Build history of the part. All positions in model axes, mm. A direction names the side the tool comes from. Give positions to 0.01 mm unless a question says otherwise; leave off trailing zeros. Write each loop counter-clockwise with the first axis right and the second up, starting at its lowest first coordinate (ties: lowest second). Pieces come first, ordered by that corner, then holes. Notation, with made-up numbers: (-32.75, -18.75) -> (-3.75, -18.75) arc R28 cw to (-3.75, 8.25) -> close; hole circle Ø10 at (-22, 25). An arc over 180 degrees is marked (long way). Put each result on its own line as item: value. Start each with the question number.
Item 1: Drill centre lines: line 1 along Y through (x, z) = (52.5, 7); line 2 along X through (y, z) = (9.5, 26.5). Where is each one in solid material? Low to high.
Item 2: Flat gauge pin, fed straight in: pin 1 Ø19 at (x, y) = (-20.5, 74) entering from +Z. Where does the tip first touch, or does it go through?
Item 3: Slice it at B-B, the plane z = 31.5. List the corners of the cut face in (x, y), plus the area to 3 significant figures.
Item 4: Slice it at C-C, the plane y = 63.5. List the corners of the cut face in (x, z), plus the area to 3 significant figures.
Item 5: Tool access for faces 1 (the cylindrical face through (-36.56, -3.39, 3.79)), 2 (the flat face through (82, -1, 25.4)), 3 (the flat face through (-1, 85.09, 15)), 4 (the flat face through (-1, -88.9, 14)): list every direction of +Z, -Z, +X, -X, +Y, -Y with a clear straight run to the whole face (end or side of a thin tool).
Item 6: Two-plate mould, pull along Y, no slides. Class faces 5 (the cylindrical face through (-87.372, 87.451, 14.13)), 6 (the cylindrical face through (-36.56, 3.39, 3.79)), 7 (the flat face through (-1, 20, 0)): pulls with the +Y half, pulls with the -Y half, needs draft (parallel to the pull), parting line crosses it, or undercut.
Item 7: Slice it at D-D, the plane z = 13. List the corners of the cut face in (x, y).
Item 8: Slice it at A-A, the plane x = -16. List the corners of the cut face in (y, z).
```python
from build123d import *

# Parameters (mm, degrees)
F0_W        = 177.8
F0_H        = 177.8
F0_W_2      = 170.18
F0_H_2      = 170.18
F1_DEPTH    = 25.4
F0_W_3      = 76.2
F0_H_3      = 9.652
F2_DEPTH    = 5.08
F3_T1_DEPTH = 5.08
F5_DEPTH    = 177.8
F6_W        = 78.74
F6_H        = 15.522254324
F7_DEPTH    = 177.801
F8_R        = 5.08
F9_R        = 2.54


# Not quite as in the source:
# - a fillet or chamfer that OpenCascade refuses, or shapes differently, is made with other operations: its cross-section is extruded or revolved along the edge and cut away or added


with BuildPart() as f1:
    # F0 (on Top) → F1 (new body)
    with BuildSketch(Plane.XY):
        Rectangle(F0_W, F0_H)
        Rectangle(F0_W_2, F0_H_2, mode=Mode.SUBTRACT)
    extrude(amount=F1_DEPTH)

    # F0 (on Top) → F2 (join)
    with BuildSketch(Plane.XY):
        Rectangle(F0_W_2, F0_H_2)
        Rectangle(F0_W_3, F0_H_3, mode=Mode.SUBTRACT)
    extrude(amount=F2_DEPTH)

    # F3: fillet of radius 5.08 on 4 edges, made by hand

    # F3_s2 → F3_t1 (join)
    with BuildSketch(Plane.XY):
        with BuildLine():
            ThreePointArc((33.02, 4.826), (36.6121024484, 3.3381024484), (38.1, -0.254))
            Line((38.1, -0.254), (38.1, 4.826))
            Line((38.1, 4.826), (33.02, 4.826))
        make_face()
        with BuildLine():
            ThreePointArc((38.1, 0.254), (36.6121024484, -3.3381024484), (33.02, -4.826))
            Line((33.02, -4.826), (38.1, -4.826))
            Line((38.1, -4.826), (38.1, 0.254))
        make_face()
        with BuildLine():
            ThreePointArc((-38.1, -0.254), (-36.6121024484, 3.3381024484), (-33.02, 4.826))
            Line((-33.02, 4.826), (-38.1, 4.826))
            Line((-38.1, 4.826), (-38.1, -0.254))
        make_face()
        with BuildLine():
            ThreePointArc((-38.1, 0.254), (-36.6121024484, -3.3381024484), (-33.02, -4.826))
            Line((-33.02, -4.826), (-38.1, -4.826))
            Line((-38.1, -4.826), (-38.1, 0.254))
        make_face()
    extrude(amount=F3_T1_DEPTH)

    # F4 (on face) → F5 (join, through all)
    with BuildSketch(Plane.YZ.offset(88.9)):
        Polygon((-50.8, 25.4), (0, 25.4), (0, 38.1), (-60.96, 38.1), align=None)
        Polygon((0, 38.1), (0, 25.4), (50.8, 25.4), (60.96, 38.1), align=None)
    extrude(amount=-F5_DEPTH)

    # F6 (on face) → F7 (cut, through all)
    with BuildSketch(Plane(origin=(0, 88.9, 0), x_dir=(-1, 0, 0), z_dir=(0, 1, 0))):
        with Locations((-39.37, 33.161127162)):
            Rectangle(F6_W, F6_H)
        with Locations((39.37, 33.161127162)):
            Rectangle(F6_W, F6_H)
    extrude(amount=-F7_DEPTH, mode=Mode.SUBTRACT)

    # F8
    f8_edges = [f1.edges().sort_by_distance(p)[0] for p in [
        (88.9, -88.9, 12.7),
        (88.9, 88.9, 12.7),
        (-88.9, 88.9, 12.7),
        (-88.9, -88.9, 12.7),
    ]]
    fillet(f8_edges, radius=F8_R)

    # F9
    f9_edges = [f1.edges().sort_by_distance(p)[0] for p in [
        (88.9, 0, 0),
        (0, 88.9, 0),
        (87.412102, -87.412102, 0),
        (87.412102, 87.412102, 0),
        (0, -88.9, 0),
        (-87.412102, -87.412102, 0),
        (-87.412102, 87.412102, 0),
        (-88.9, 0, 0),
        (0, -4.826, 0),
        (-36.521148, -3.42681, 0),
        (-36.521148, 3.42681, 0),
        (0, 4.826, 0),
        (36.521148, 3.42681, 0),
        (36.521148, -3.42681, 0),
    ]]
    fillet(f9_edges, radius=F9_R)


solid = f1.part
```
Values follow:
1. line 1: -88.9 to -85.09, 85.09 to 88.9
1. line 2: -88.9 to -78.74, 78.74 to 88.9
2. pin 1: z = 5.08
3. outline: (-88.9, -55.68) -> (-78.74, -55.68) -> (-78.74, 55.68) -> (-88.9, 55.68) -> close; (78.74, -55.68) -> (88.9, -55.68) -> (88.9, 55.68) -> (78.74, 55.68) -> close
3. area: 2,260 mm2
4. outline: (-88.9, 2.54) arc R2.54 ccw to (-86.36, 0) -> (86.36, 0) arc R2.54 ccw to (88.9, 2.54) -> (88.9, 25.4) -> (85.09, 25.4) -> (85.09, 5.08) -> (-85.09, 5.08) -> (-85.09, 25.4) -> (-88.9, 25.4) -> close
4. area: 1,060 mm2
5. face 1: +Z, -Z
5. face 2: none
5. face 3: +Z
5. face 4: +Z, -Z, +X, -X, -Y
6. face 5: pulls with the +Y half
6. face 6: undercut
6. face 7: needs draft
7. outline: (-88.9, -83.82) arc R5.08 ccw to (-83.82, -88.9) -> (83.82, -88.9) arc R5.08 ccw to (88.9, -83.82) -> (88.9, 83.82) arc R5.08 ccw to (83.82, 88.9) -> (-83.82, 88.9) arc R5.08 ccw to (-88.9, 83.82) -> close; hole (-85.09, -85.09) -> (85.09, -85.09) -> (85.09, 85.09) -> (-85.09, 85.09) -> close
8. outline: (-88.9, 2.54) arc R2.54 ccw to (-86.36, 0) -> (-7.37, 0) arc R2.54 ccw to (-4.83, 2.54) -> (-4.83, 5.08) -> (-85.09, 5.08) -> (-85.09, 25.4) -> (-88.9, 25.4) -> close; (4.83, 2.54) arc R2.54 ccw to (7.37, 0) -> (86.36, 0) arc R2.54 ccw to (88.9, 2.54) -> (88.9, 25.4) -> (85.09, 25.4) -> (85.09, 5.08) -> (4.83, 5.08) -> close
